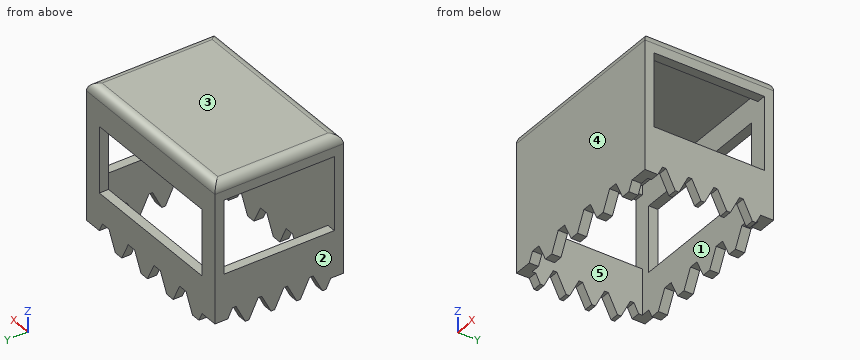
```python
from build123d import *

# Parameters (mm, degrees)
SKETCH1_W               = 100
SKETCH1_H               = 70
BOSS_EXTRUDE1_DEPTH     = 80
FILLET2_R               = 5
CUT_EXTRUDE1_START      = -5
SKETCH3_W               = 90
SKETCH3_H               = 60
CUT_EXTRUDE1_DEPTH      = 75
SKETCH2_W               = 40
SKETCH2_H               = 60
CUT_EXTRUDE2_DEPTH      = 5
SKETCH4_W               = 40
SKETCH4_H               = 60
CUT_EXTRUDE3_DEPTH      = 5
CUT_EXTRUDE4_START      = -5
CUT_EXTRUDE4_DEPTH      = 5
CUT_EXTRUDE5_START      = -5
CUT_EXTRUDE5_DEPTH      = 5
CUT_EXTRUDE6_DEPTH      = 118.633373344
CUT_EXTRUDE6_DEPTH_BACK = 5
CUT_EXTRUDE7_DEPTH      = 118.633373344
CUT_EXTRUDE7_DEPTH_BACK = 5
SKETCH9_W               = 80
SKETCH9_H               = 36
CUT_EXTRUDE8_DEPTH      = 5


# Read off the part's stored shape, not the designer's step: Cut-Extrude4, Cut-Extrude5
with BuildPart() as part:
    # Sketch1 → Boss-Extrude1 (new body)
    with BuildSketch(Plane.XY):
        with Locations((-0.374701232, -1.49844749)):
            Rectangle(SKETCH1_W, SKETCH1_H)
    extrude(amount=-BOSS_EXTRUDE1_DEPTH)

    # Fillet2
    fillet2_edges = [part.edges().sort_by_distance(p)[0] for p in [
        (-0.374701232, 33.50155251, 0),
        (49.625298768, -1.49844749, 0),
        (-0.374701232, -36.49844749, 0),
        (-50.374701232, -1.49844749, 0),
    ]]
    fillet(fillet2_edges, radius=FILLET2_R)

    # Sketch3 → Cut-Extrude1 (cut)
    with BuildSketch(Plane.XY.offset(CUT_EXTRUDE1_START)):
        with Locations((-0.374701232, -1.49844749)):
            Rectangle(SKETCH3_W, SKETCH3_H)
    extrude(amount=-CUT_EXTRUDE1_DEPTH, mode=Mode.SUBTRACT)

    # Sketch2 → Cut-Extrude2 (cut)
    with BuildSketch(Plane(origin=(49.625298768, 0, 0), x_dir=(0, 0, -1), z_dir=(1, 0, 0))):
        with Locations((30, -1.49844749)):
            Rectangle(SKETCH2_W, SKETCH2_H)
    extrude(amount=-CUT_EXTRUDE2_DEPTH, mode=Mode.SUBTRACT)

    # Sketch4 → Cut-Extrude3 (cut)
    with BuildSketch(Plane.ZY.offset(50.374701232)):
        with Locations((-30, -1.49844749)):
            Rectangle(SKETCH4_W, SKETCH4_H)
    extrude(amount=-CUT_EXTRUDE3_DEPTH, mode=Mode.SUBTRACT)

    # Cut-Extrude4 outline → Cut-Extrude4 (cut)
    with BuildSketch(Plane(origin=(49.625298768, 0, 0), x_dir=(0, 0, -1), z_dir=(1, 0, 0)).offset(CUT_EXTRUDE4_START)):
        Polygon((80, -19.99844749), (70, -24.99844749), (70, -26.99844749), (75, -29.49844749), (75, -36.49844749), (80, -36.49844749), align=None)
        Polygon((75, 26.50155251), (80, 24.00155251), (80, 33.50155251), (75, 33.50155251), align=None)
        Polygon((70, 15.00155251), (80, 10.00155251), (80, 22.00155251), (70, 17.00155251), align=None)
        Polygon((70, 1.00155251), (80, -3.99844749), (80, 8.00155251), (70, 3.00155251), align=None)
        Polygon((70, -12.99844749), (80, -17.99844749), (80, -5.99844749), (70, -10.99844749), align=None)
    extrude(amount=CUT_EXTRUDE4_DEPTH, mode=Mode.SUBTRACT)

    # Cut-Extrude5 outline → Cut-Extrude5 (cut)
    with BuildSketch(Plane.ZY.offset(50.374701232).offset(CUT_EXTRUDE5_START)):
        Polygon((-80, 17.00155251), (-70, 22.00155251), (-70, 24.00155251), (-75, 26.50155251), (-75, 33.50155251), (-80, 33.50155251), align=None)
        Polygon((-75, -29.49844749), (-80, -26.99844749), (-80, -36.49844749), (-75, -36.49844749), align=None)
        Polygon((-70, -17.99844749), (-80, -12.99844749), (-80, -24.99844749), (-70, -19.99844749), align=None)
        Polygon((-70, -3.99844749), (-80, 1.00155251), (-80, -10.99844749), (-70, -5.99844749), align=None)
        Polygon((-70, 10.00155251), (-80, 15.00155251), (-80, 3.00155251), (-70, 8.00155251), align=None)
    extrude(amount=CUT_EXTRUDE5_DEPTH, mode=Mode.SUBTRACT)

    # Sketch7 → Cut-Extrude6 (cut, two sides: drawn at the far end of the back side and taken through both)
    with BuildSketch(Plane(origin=(0, 33.50155251, 0), x_dir=(1, 0, 0), z_dir=(0, 1, 0)).offset(-CUT_EXTRUDE6_DEPTH_BACK)):
        Polygon((-297.449069971, 75), (-45.374701232, 75), (-40.374701232, 75), (-37.874701232, 80), (-32.874701232, 80), (-27.874701232, 70), (-22.874701232, 70), (-17.874701232, 80), (-12.874701232, 80), (-7.874701232, 70), (-2.874701232, 70), (2.125298768, 80), (7.125298768, 80), (12.125298768, 70), (17.125298768, 70), (22.125298768, 80), (27.125298768, 80), (32.125298768, 70), (37.125298768, 70), (39.625298768, 75), (44.625298768, 75), (296.699667506, 75), (296.699667506, 579.148737476), (-297.449069971, 579.148737476), align=None)
    extrude(amount=CUT_EXTRUDE6_DEPTH + CUT_EXTRUDE6_DEPTH_BACK, mode=Mode.SUBTRACT)

    # Sketch8 → Cut-Extrude7 (cut, two sides: drawn at the far end of the back side and taken through both)
    with BuildSketch(Plane.XZ.offset(36.49844749).offset(-CUT_EXTRUDE7_DEPTH_BACK)):
        Polygon((-297.449069971, -75), (-45.374701232, -75), (-40.374701232, -75), (-37.874701232, -70), (-32.874701232, -70), (-27.874701232, -80), (-22.874701232, -80), (-17.874701232, -70), (-12.874701232, -70), (-7.874701232, -80), (-2.874701232, -80), (2.125298768, -70), (7.125298768, -70), (12.125298768, -80), (17.125298768, -80), (22.125298768, -70), (27.125298768, -70), (32.125298768, -80), (37.125298768, -80), (39.625298768, -75), (44.625298768, -75), (296.699667506, -75), (296.699667506, -579.148737476), (-297.449069971, -579.148737476), align=None)
    extrude(amount=CUT_EXTRUDE7_DEPTH + CUT_EXTRUDE7_DEPTH_BACK, mode=Mode.SUBTRACT)

    # Sketch9 → Cut-Extrude8 (cut)
    with BuildSketch(Plane(origin=(0, 33.50155251, 0), x_dir=(1, 0, 0), z_dir=(0, 1, 0))):
        with Locations((-0.374701232, 36.675611874)):
            Rectangle(SKETCH9_W, SKETCH9_H)
    extrude(amount=-CUT_EXTRUDE8_DEPTH, mode=Mode.SUBTRACT)


solid = part.part
```
The listing builds one solid part. Answer for the finished solid, in the listing's coordinates (mm). Face numbers are marked on the shaded views. A direction names the side the tool comes from. Give positions to 0.01 mm unless a question says otherwise; leave off trailing zeros. Order: outer loops, then holes, each group sorted by start corner. A loop starts at its lowest first (then second) coordinate and runs counter-clockwise, first axis right, second up.
Item 1: Given pin 1 Ø1.5 at (x, y) = (-6, 30) entering from -Z; pin 2 Ø1 at (x, z) = (-2.5, -38) entering from +Y; pin 3 Ø4 at (x, y) = (-36, -33) entering from -Z; pin 4 Ø5.5 at (x, y) = (-49, 0) entering from -Z, each flat-ended and moving along its own axis, determine where each tip first touches the part or whether it passes through.
From the geometry:
pin 1: stops at z = -70
pin 2: stops at y = -31.5
pin 3: stops at z = -70.25
pin 4: stops at z = -80
Item 2: Which of the six approach directions +Z, -Z, +X, -X, +Y, -Y give full straight-line access (tool end or side, diameter ignored) to the marked faces 4 and 5?
From the geometry:
face 4: +Z, -Z, +X, -X, -Y
face 5: -Z
Item 3: Find the intervals of material crossed by probe 1 along X at (y, z) = (15.5, -58); probe 2 along Y at (x, z) = (19.5, -59); probe 3 along Z at (x, y) = (-23, 1), in increasing order.
From the geometry:
probe 1: x = -50.37 to -45.37, 44.63 to 49.63
probe 2: y = -36.5 to -31.5, 28.5 to 33.5
probe 3: z = -5 to 0
Item 4: The part is cut by section A-A, the plane z = -27. Give the vertices of the cut face in (x, y), and give its area (3 significant figures).
From the geometry:
outline: (-50.37, -36.5) - (49.63, -36.5) - (49.63, -31.5) - (-50.37, -31.5) - close; (-50.37, 28.5) - (-40.37, 28.5) - (-40.37, 33.5) - (-50.37, 33.5) - close; (39.63, 28.5) - (49.63, 28.5) - (49.63, 33.5) - (39.63, 33.5) - close
area: 600 mm2
Item 5: The part is cut by section C-C, the plane z = -68.5. Give the vertices of the cut face in (x, y), and give its area (3 significant figures).
From the geometry:
outline: (-50.37, -36.5) - (49.63, -36.5) - (49.63, 33.5) - (-50.37, 33.5) - close; hole (-45.37, -31.5) - (44.63, -31.5) - (44.63, 28.5) - (-45.37, 28.5) - close
area: 1,600 mm2
Item 6: The part is cut by section B-B, the plane x = -15. Give the vertices of the cut face in (y, z), and give its area (3 significant figures).
From the geometry:
outline: (-36.5, -70) - (-31.5, -70) - (-31.5, -5) - (28.5, -5) - (28.5, -18.68) - (33.5, -18.68) - (33.5, -5) arc R5 ccw to (28.5, 0) - (-31.5, 0) arc R5 ccw to (-36.5, -5) - close; (28.5, -80) - (33.5, -80) - (33.5, -54.68) - (28.5, -54.68) - close
area: 859 mm2
Item 7: The part is cut by section D-D, the plane y = -23. Give the vertices of the cut face in (x, z).
From the geometry:
outline: (-50.37, -76) - (-45.37, -76) - (-45.37, -50) - (-50.37, -50) - close; (-50.37, -10) - (-45.37, -10) - (-45.37, -5) - (44.63, -5) - (44.63, -10) - (49.63, -10) - (49.63, -5) arc R5 ccw to (44.63, 0) - (-45.37, 0) arc R5 ccw to (-50.37, -5) - close; (44.63, -74) - (49.63, -74) - (49.63, -50) - (44.63, -50) - close
Item 8: For a pull along X with two mould halves and no side action, classify the marked faces 1, 2 and 3 as pulls with the +X half, pulls with the -X half, needs draft (parallel to the pull), parting line crosses it, or undercut.
From the geometry:
face 1: undercut
face 2: pulls with the -X half
face 3: needs draft
